Here's how the part is built. I have some questions about the finished solid (model axes, mm). Face numbers are marked on the shaded views. Coordinates: 2 decimals unless noted, no trailing zeros. Write each loop counter-clockwise with the first axis right and the second up, starting at its lowest first coordinate (ties: lowest second). Pieces come first, ordered by that corner, then holes. Notation, with made-up numbers: M 37.25,55.5 L 81.25,55.5 A8 cw 81.25,67.5 Z; hole C 30.25,74 d8. An arc over 180 degrees is marked long. Use a Markdown table: item, result.
Autodesk Inventor part; units mm, degrees
ref_plane "工作平面1" through (0, 0, 2) normal (0, 0, 1) x (1, 0, 0)
ref_plane "工作平面2" through (11.25, -28.7256, 2) normal (0.3647, -0.9311, 0) x (0.9311, 0.3647, 0)
ref_plane "工作平面3" through (-11.25, -28.7256, 2) normal (-0.3647, -0.9311, 0) x (0.9311, -0.3647, 0)
sketch "草圖1" plane through (0, 0, 0) normal (0, 0, 1) x (1, 0, 0)
  circle A0 centre (0, 0) radius 30.85
  circle A1 centre (0, 0) radius 25.95
  dimension "d0" = 61.7
  dimension "d3" = 51.9
extrude "擠出1" add sketch "草圖1" along normal blind 4
sketch "草圖2" plane through (0, 0, 4) normal (0, 0, 1) x (1, 0, 0)
  circle A0 centre (0, 0) radius 25.95
  circle A1 centre (0, 0) radius 30.85
  line L0 (0, 0) -> (0, 30.85)
  line L1 (11, 28.8223) -> (11, 23.5032)
  line L2 (-11, 28.8223) -> (-11, 23.5032)
  dimension "d6" = 22
extrude "擠出2" cut sketch "草圖2" against normal blind 2.5 contours A0 L0 A1 L1 | L2 A1 L0 A0
ref_plane "工作平面1" through (0, 0, 2) normal (0, 0, 1) x (1, 0, 0)
sketch "草圖3" plane through (0, 0, 2) normal (0, 0, 1) x (1, 0, 0)
  line L0 (0, 0) -> (0, -42.4806)
  line L1 (0, 0) -> (-11.25, -28.7256)
  line L2 (0, 0) -> (11.25, -28.7256)
  arc A0 (-11, 28.8223) -> (11, 28.8223) centre (0, 0) ccw
  line L3 (-11.25, -28.7256) -> (11.25, -28.7256)
  dimension "d9" = 22.5
ref_plane "工作平面2" through (11.25, -28.7256, 2) normal (0.3647, -0.9311, 0) x (0.9311, 0.3647, 0)
ref_plane "工作平面3" through (-11.25, -28.7256, 2) normal (-0.3647, -0.9311, 0) x (0.9311, -0.3647, 0)
sketch "草圖4" plane through (11.25, -28.7256, 2) normal (0.3647, -0.9311, 0) x (0.9311, 0.3647, 0)
  point P0 (0, -2)
  point P1 (0, 0)
hole "孔1" at (11.25, -28.7256, 2) direction (-0.3647, 0.9311, 0) diameter 2 depth 2.5 tip angle 118
sketch "草圖5" plane through (-11.25, -28.7256, 2) normal (-0.3647, -0.9311, 0) x (0.9311, -0.3647, 0)
  point P0 (0, -2)
  point P1 (0, 0)
hole "孔2" at (-11.25, -28.7256, 2) direction (0.3647, 0.9311, 0) diameter 2 depth 2.5 tip angle 118
chamfer "倒角1" distance 0.5 angle 45 6 edges at (-13.9275, -21.8958, 4) (21.8958, 13.9275, 4) (-25.95, 0, 0) (-17.4982, -25.4074, 4) (25.4074, 17.4982, 4) (-30.85, 0, 0)
properties part number "KE-SP-02-P1"
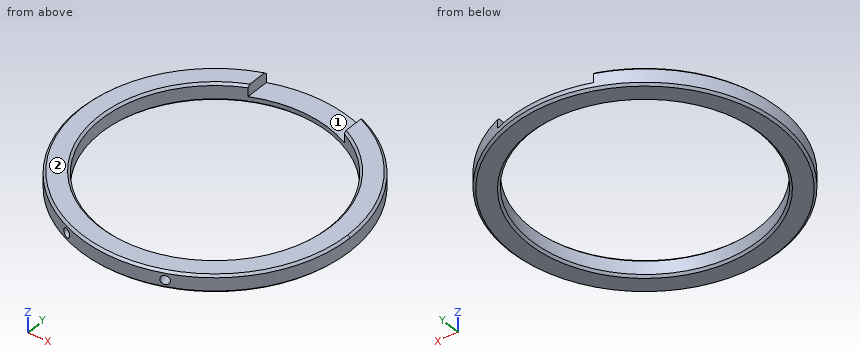
1. I need wall thicknesses on probe 1 along Y at (x, z) = (0, 1.2); probe 2 along Y at (x, z) = (5.5, 1.1). Which ranges of each line are inside material? Lowest first, please.
Answers follow:
| item | result |
|---|---|
| probe 1 | y = -30.85 to -25.95, 25.95 to 30.85 |
| probe 2 | y = -30.36 to -25.36, 25.36 to 30.36 |
2. Will these pins go through, and if not, where does the flat tip stop? pin 1 Ø3.5 at (x, y) = (-1.5, 28.5) entering from +Z; pin 2 Ø8 at (x, y) = (-19, -15) entering from +Z; pin 3 Ø1.5 at (x, z) = (14, 1) entering from +Y; pin 4 Ø0.8 at (y, z) = (27, 3.5) entering from +X.
Answers follow:
| item | result |
|---|---|
| pin 1 | stops at z = 1.5 |
| pin 2 | stops at z = 4 |
| pin 3 | stops at y = 27.86 |
| pin 4 | stops at x = 15.63 |
3. Suppose I cut it at A-A on x = 0. Write out the boundary of the cut face in (y, z), and give its area (3 significant figures).
Answers follow:
| item | result |
|---|---|
| outline | M -30.85,0.5 L -30.35,0 L -26.45,0 L -25.95,0.5 L -25.95,3.5 L -26.45,4 L -30.35,4 L -30.85,3.5 Z; M 25.95,0.5 L 26.45,0 L 30.35,0 L 30.85,0.5 L 30.85,1.5 L 25.95,1.5 Z |
| area | 26.2 mm2 |
4. We'd pull the mould along X, two halves only. Please class the marked faces 1 and 2: +X half, -X half, draft (parallel to the pull), parting line (faces both ways), or undercut.
Answers follow:
| item | result |
|---|---|
| face 1 | undercut |
| face 2 | draft |
